Here's how the part is built. I have some questions about the finished solid (model axes, mm). Round coordinates to 2 decimals unless told otherwise and drop trailing zeros. Order: outer loops, then holes, each group sorted by start corner. A loop starts at its lowest first (then second) coordinate and runs counter-clockwise, first axis right, second up. Notation, with made-up numbers: M -21.5,57 L -7.5,57 A25 ccw -7.5,71 Z; hole C -34.5,50 d5. An arc over 180 degrees is marked long. Answer as CSV lines item,"result". Start each with the question number.
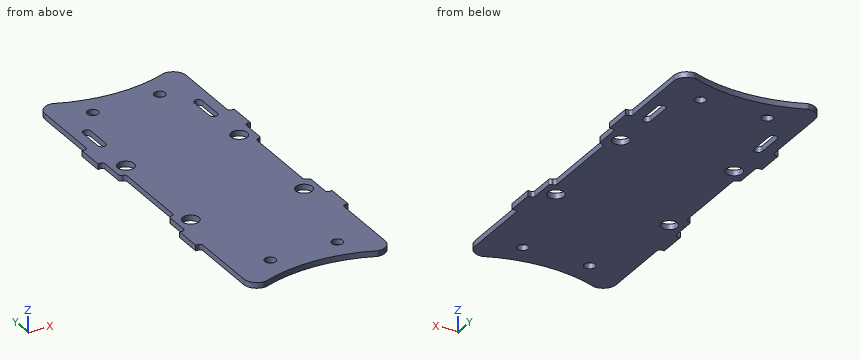
```python
from build123d import *

# Parameters (mm, degrees)
F0_R     = 1.5
F0_R_2   = 2.225
F1_DEPTH = 1.5


# Not quite as in the source:
# - ends of sketch curves that miss each other by under 0.0002 mm in the source are joined


with BuildPart() as f1:
    # F0 (on Top) → F1 (new body)
    with BuildSketch(Plane.XY):
        with BuildLine():
            ThreePointArc((19.75, -19.25), (19.2196699141, -19.0303300859), (19, -18.5))
            Line((19, -18.5), (19, -12.25))
            ThreePointArc((19, -12.25), (18.7803300859, -11.7196699141), (18.25, -11.5))
            ThreePointArc((18.25, -11.5), (17.7196699141, -11.2803300859), (17.5, -10.75))
            Line((17.5, -10.75), (17.5, 10.75))
            ThreePointArc((17.5, 10.75), (17.7196699141, 11.2803300859), (18.25, 11.5))
            ThreePointArc((18.25, 11.5), (18.7803300859, 11.7196699141), (19, 12.25))
            Line((19, 12.25), (19, 18.5))
            ThreePointArc((19, 18.5), (19.2196699141, 19.0303300859), (19.75, 19.25))
            Line((19.75, 19.25), (20.5, 19.25))
            Line((20.5, 19.25), (20.5, 26.75))
            Line((20.5, 26.75), (19.75, 26.75))
            ThreePointArc((19.75, 26.75), (19.2196699141, 26.9696699141), (19, 27.5))
            Line((19, 27.5), (19, 46.75))
            ThreePointArc((19, 46.75), (17.9748737342, 49.2248737342), (15.5, 50.25))
            Line((15.5, 50.25), (15.167259, 50.25))
            ThreePointArc((15.167259, 50.25), (0, 47.25), (-15.1672590116, 50.2499999718))
            Line((-15.1672590116, 50.2499999718), (-15.5, 50.25))
            ThreePointArc((-15.5, 50.25), (-17.9748737342, 49.2248737342), (-19, 46.75))
            Line((-19, 46.75), (-19, 27.5))
            ThreePointArc((-19, 27.5), (-19.2196699141, 26.9696699141), (-19.75, 26.75))
            Line((-19.75, 26.75), (-20.5, 26.75))
            Line((-20.5, 26.75), (-20.5, 19.25))
            Line((-20.5, 19.25), (-19.75, 19.25))
            ThreePointArc((-19.75, 19.25), (-19.2196699141, 19.0303300859), (-19, 18.5))
            Line((-19, 18.5), (-19, 12.25))
            ThreePointArc((-19, 12.25), (-18.7803300859, 11.7196699141), (-18.25, 11.5))
            ThreePointArc((-18.25, 11.5), (-17.7196699141, 11.2803300859), (-17.5, 10.75))
            Line((-17.5, 10.75), (-17.5, -10.75))
            ThreePointArc((-17.5, -10.75), (-17.7196699141, -11.2803300859), (-18.25, -11.5))
            ThreePointArc((-18.25, -11.5), (-18.7803300859, -11.7196699141), (-19, -12.25))
            Line((-19, -12.25), (-19, -18.5))
            ThreePointArc((-19, -18.5), (-19.2196699141, -19.0303300859), (-19.75, -19.25))
            Line((-19.75, -19.25), (-20.5, -19.25))
            Line((-20.5, -19.25), (-20.5, -26.75))
            Line((-20.5, -26.75), (-19.75, -26.75))
            ThreePointArc((-19.75, -26.75), (-19.2196699141, -26.9696699141), (-19, -27.5))
            Line((-19, -27.5), (-19, -46.75))
            ThreePointArc((-19, -46.75), (-17.9748737342, -49.2248737342), (-15.5, -50.25))
            Line((-15.5, -50.25), (-15.167259, -50.25))
            ThreePointArc((-15.167259, -50.25), (0, -47.249999), (15.1672593636, -50.2499991168))
            Line((15.1672593636, -50.2499991168), (15.5, -50.25))
            ThreePointArc((15.5, -50.25), (17.9748737342, -49.2248737342), (19, -46.75))
            Line((19, -46.75), (19, -27.5))
            ThreePointArc((19, -27.5), (19.2196699141, -26.9696699141), (19.75, -26.75))
            Line((19.75, -26.75), (20.5, -26.75))
            Line((20.5, -26.75), (20.5, -19.25))
            Line((20.5, -19.25), (19.75, -19.25))
        make_face()
        with Locations((-9, -41.75)):
            Circle(F0_R, mode=Mode.SUBTRACT)
        with Locations((-15.25, -15.25)):
            Circle(F0_R_2, mode=Mode.SUBTRACT)
        with Locations((9, -41.75)):
            Circle(F0_R, mode=Mode.SUBTRACT)
        with Locations((15.25, -15.25)):
            Circle(F0_R_2, mode=Mode.SUBTRACT)
        with Locations((-15.25, 15.25)):
            Circle(F0_R_2, mode=Mode.SUBTRACT)
        with BuildLine():
            ThreePointArc((-16.1, 34.033918), (-15, 35.133918), (-13.9, 34.033918))
            Line((-13.9, 34.033918), (-13.9, 27.033918))
            ThreePointArc((-13.9, 27.033918), (-15, 25.933918), (-16.1, 27.033918))
            Line((-16.1, 27.033918), (-16.1, 34.033918))
        make_face(mode=Mode.SUBTRACT)
        with Locations((-9, 41.75)):
            Circle(F0_R, mode=Mode.SUBTRACT)
        with Locations((15.25, 15.25)):
            Circle(F0_R_2, mode=Mode.SUBTRACT)
        with Locations((9, 41.75)):
            Circle(F0_R, mode=Mode.SUBTRACT)
        with BuildLine():
            ThreePointArc((13.9, 34.033918), (15, 35.133918), (16.1, 34.033918))
            Line((16.1, 34.033918), (16.1, 27.033918))
            ThreePointArc((16.1, 27.033918), (15, 25.933918), (13.9, 27.033918))
            Line((13.9, 27.033918), (13.9, 34.033918))
        make_face(mode=Mode.SUBTRACT)
    extrude(amount=F1_DEPTH)


solid = f1.part
```
Item 1: If I drill on line 1 along X through (y, z) = (15, 1.1); line 2 along Y through (x, z) = (-15.5, 0.3); line 3 along X through (y, z) = (-17, 0.1), over which ranges is the centre line in solid material (lowest first)?
Item 2: If we section it at B-B on x = -9: Please give me the cut outline in (y, z).
Item 3: If we section it at C-C on y = -29.5: Please give me the cut outline in (x, z).
Item 4: If we section it at D-D on z = 0.55: Count the separate pieces of the cut face and the enclosed holes in it, and give its area (3 significant figures).
Item 5: For P1, Ø0.8, axis at y = 31.5, z = 1, coming from the -X side; P2, Ø0.8, axis at x = 20.5, z = 0.5, coming from the +Y side, each with a flat end and sliding along its axis, tell me the tip position at first contact or that it passes through.
Item 6: If we section it at A-A on y = 41.75: Please give me the cut outline in (x, z).
Geometry says:
1,line 1,"-19 to -17.46, -13.04 to 13.04, 17.46 to 19"
1,line 2,"-50.25 to -17.46, -13.04 to 13.04, 17.46 to 26.05, 35.01 to 50.25"
1,line 3,"-19 to -16.62, -13.88 to 13.88, 16.62 to 19"
2,outline,"M -48.28,0 L -43.25,0 L -43.25,1.5 L -48.28,1.5 Z; M -40.25,0 L 40.25,0 L 40.25,1.5 L -40.25,1.5 Z; M 43.25,0 L 48.28,0 L 48.28,1.5 L 43.25,1.5 Z"
3,outline,"M -19,0 L 19,0 L 19,1.5 L -19,1.5 Z"
4,separate pieces,"1"
4,enclosed holes,"10"
4,area,"3,530 mm²"
5,P1,"x = -19"
5,P2,"y = 26.75"
6,outline,"M -19,0 L -10.5,0 L -10.5,1.5 L -19,1.5 Z; M -7.5,0 L 7.5,0 L 7.5,1.5 L -7.5,1.5 Z; M 10.5,0 L 19,0 L 19,1.5 L 10.5,1.5 Z"
